from build123d import *

# Parameters (mm, degrees)
SKETCH_1_R          = 18
EXTRUDE_1_DEPTH     = 32.5
SKETCH_1_3_W        = 42
SKETCH_1_3_H        = 42
SKETCH_1_3_R        = 18
EXTRUDE_2_DEPTH     = 2.5
FILLET_1_R          = 3
SKETCH_4_R          = 1.6
CUT_EXTRUDE_1_DEPTH = 2.5
SKETCH_5_R          = 11
EXTRUDE_3_DEPTH     = 3.5
EXTRUDE_4_DEPTH     = 15
SKETCH_7_R          = 11
CUT_EXTRUDE_2_DEPTH = 25


with BuildPart() as part:
    # Sketch 1 → Extrude 1 (new body)
    with BuildSketch(Plane.XY):
        Circle(SKETCH_1_R)
    extrude(amount=EXTRUDE_1_DEPTH)

    # Sketch 1_3 → Extrude 2 (add)
    with BuildSketch(Plane.XY):
        Rectangle(SKETCH_1_3_W, SKETCH_1_3_H)
        with Locations(Location((0, 0, 0), (0, 0, 180))):
            Circle(SKETCH_1_3_R, mode=Mode.SUBTRACT)
    extrude(amount=EXTRUDE_2_DEPTH)

    # Fillet 1
    fillet_1_edges = [part.edges().sort_by_distance(p)[0] for p in [
        (21, -21, 1.25),
        (21, 21, 1.25),
        (-21, 21, 1.25),
        (-21, -21, 1.25),
    ]]
    fillet(fillet_1_edges, radius=FILLET_1_R)

    # Sketch 4 → Cut-Extrude 1 (cut)
    with BuildSketch(Plane(origin=(0, 0, 0), x_dir=(-1, 0, 0), z_dir=(0, 0, -1))):
        with Locations((-15.5, 15.5)):
            Circle(SKETCH_4_R)
        with Locations((-15.5, -15.5)):
            Circle(SKETCH_4_R)
        with Locations((15.5, -15.5)):
            Circle(SKETCH_4_R)
        with Locations((15.5, 15.5)):
            Circle(SKETCH_4_R)
    extrude(amount=-CUT_EXTRUDE_1_DEPTH, mode=Mode.SUBTRACT)

    # Sketch 5 → Extrude 3 (add)
    with BuildSketch(Plane.XY.offset(32.5)):
        Circle(SKETCH_5_R)
    extrude(amount=EXTRUDE_3_DEPTH)

    # Sketch 6 → Extrude 4 (add)
    with BuildSketch(Plane.XY.offset(36)):
        with BuildLine():
            Line((-2.645751311, -3), (2.645751311, -3))
            ThreePointArc((2.645751311, -3), (4, 0), (2.645751311, 3))
            Line((2.645751311, 3), (-2.645751311, 3))
            ThreePointArc((-2.645751311, 3), (-4, 0), (-2.645751311, -3))
        make_face()
    extrude(amount=EXTRUDE_4_DEPTH)

    # Sketch 7 → Cut-Extrude 2 (cut)
    with BuildSketch(Plane(origin=(0, 0, 0), x_dir=(-1, 0, 0), z_dir=(0, 0, -1))):
        with Locations(Location((0, 0, 0), (0, 0, 180))):
            Circle(SKETCH_7_R)
    extrude(amount=-CUT_EXTRUDE_2_DEPTH, mode=Mode.SUBTRACT)


solid = part.part
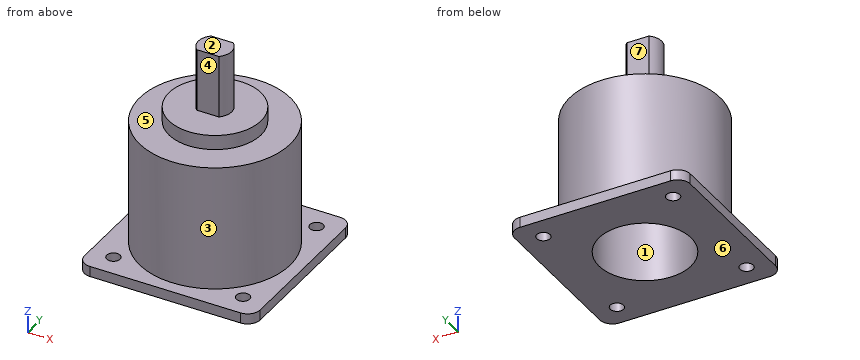
The listing builds one solid part. Answer for the finished solid, in the listing's coordinates (mm). Face numbers are marked on the shaded views. A direction names the side the tool comes from. Round coordinates to 2 decimals unless told otherwise and drop trailing zeros. Order: outer loops, then holes, each group sorted by start corner. A loop starts at its lowest first (then second) coordinate and runs counter-clockwise, first axis right, second up. Notation, with made-up numbers: (78, 17) -> (126, 17) arc R15 cw to (126, 26) -> close; hole circle Ø1 at (23, 7). An arc over 180 degrees is marked (long way). One line per item, written item: value.
Item 1: For a pull along X with two mould halves and no side action, classify the marked faces 1, 2 and 3 as released by +X, released by -X, zero draft, split by the parting line, or undercut.
Taken from the geometry:
face 1: undercut
face 2: zero draft
face 3: split by the parting line
Item 2: Find section B-B, the plane z = 13.5. Give the vertices of the cut face in (x, y), then the cut area to 3 significant figures.
Taken from the geometry:
outline: circle Ø36 at (0, 0); hole circle Ø22 at (0, 0)
area: 638 mm2
Item 3: For the marked faces 4, 5, 6 and 7, determine the directions among +Z, -Z, +X, -X, +Y, -Y from which every point of the face is accessible in a straight line to the end or side of a thin tool.
Taken from the geometry:
face 4: +Z, +X, -X, -Y
face 5: +Z
face 6: -Z, +X, -X, +Y, -Y
face 7: +Z, +X, -X, +Y
Item 4: Straight lines are drawn through the part: L1, parallel to Y at x = 15, z = 1; L2, parallel to Y at x = 15.5, z = 1.7. For each, find the intervals that lie inside material, in ascending order.
Taken from the geometry:
L1: y = -21 to -17.02, -13.98 to 13.98, 17.02 to 21
L2: y = -21 to -17.1, -13.9 to 13.9, 17.1 to 21
Item 5: Given P1, Ø3, axis at x = 5, y = -9, coming from the +Z side; P2, Ø1.5, axis at x = 7, y = -16, coming from the +Z side; P3, Ø10, axis at x = 14, z = 37, coming from the -Y side, each flat-ended and moving along its own axis, determine where each tip first touches the part or whether it passes through.
Taken from the geometry:
P1: stops at z = 36
P2: stops at z = 32.5
P3: stops at y = -13.57
Item 6: Find section A-A, the plane y = -15.5. Give the vertices of the cut face in (x, z), then the cut area to 3 significant figures.
Taken from the geometry:
outline: (-21, 0) -> (-17.1, 0) -> (-17.1, 2.5) -> (-21, 2.5) -> close; (-13.9, 0) -> (13.9, 0) -> (13.9, 2.5) -> (9.15, 2.5) -> (9.15, 32.5) -> (-9.15, 32.5) -> (-9.15, 2.5) -> (-13.9, 2.5) -> close; (17.1, 0) -> (21, 0) -> (21, 2.5) -> (17.1, 2.5) -> close
area: 638 mm2
Item 7: Find section D-D, the plane y = 0. Give the vertices of the cut face in (x, z), then the cut area to 3 significant figures.
Taken from the geometry:
outline: (-21, 0) -> (-11, 0) -> (-11, 25) -> (11, 25) -> (11, 0) -> (21, 0) -> (21, 2.5) -> (18, 2.5) -> (18, 32.5) -> (11, 32.5) -> (11, 36) -> (4, 36) -> (4, 51) -> (-4, 51) -> (-4, 36) -> (-11, 36) -> (-11, 32.5) -> (-18, 32.5) -> (-18, 2.5) -> (-21, 2.5) -> close
area: 832 mm2
Item 8: Find section C-C, the plane x = 0. Give the vertices of the cut face in (y, z).
Taken from the geometry:
outline: (-21, 0) -> (-11, 0) -> (-11, 25) -> (11, 25) -> (11, 0) -> (21, 0) -> (21, 2.5) -> (18, 2.5) -> (18, 32.5) -> (11, 32.5) -> (11, 36) -> (3, 36) -> (3, 51) -> (-3, 51) -> (-3, 36) -> (-11, 36) -> (-11, 32.5) -> (-18, 32.5) -> (-18, 2.5) -> (-21, 2.5) -> close
